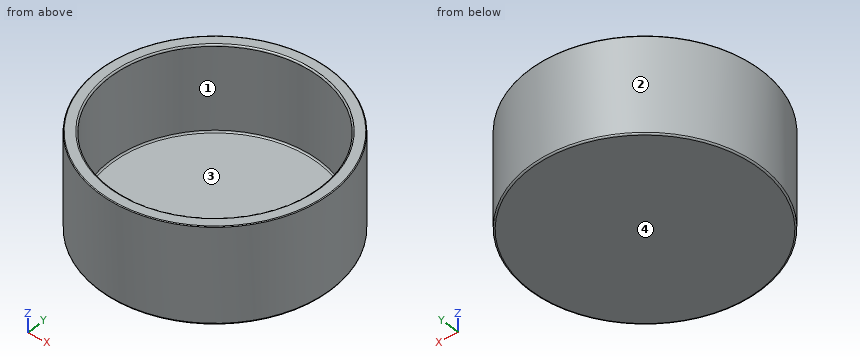
```python
from build123d import *

# Parameters (mm, degrees)
F0_R     = 31.25
F1_DEPTH = 3
F2_R     = 31.25
F2_R_2   = 28.25
F3_DEPTH = 23
F4_R     = 0.4
F5_R     = 0.2


with BuildPart() as f1:
    # F0 (on Top) → F1 (new body)
    with BuildSketch(Plane.XY):
        Circle(F0_R)
    extrude(amount=F1_DEPTH)

    # F2 (on face) → F3 (join)
    with BuildSketch(Plane.XY.offset(3)):
        Circle(F2_R)
        Circle(F2_R_2, mode=Mode.SUBTRACT)
    extrude(amount=F3_DEPTH)

    # F4
    f4_edges = [f1.edges().sort_by_distance(p)[0] for p in [
        (-28.25, 0, 26),
        (-28.25, 0, 3),
        (-31.25, 0, 0),
    ]]
    fillet(f4_edges, radius=F4_R)

    # F5
    f5_edges = [f1.edges().sort_by_distance(p)[0] for p in [
        (-31.25, 0, 26),
    ]]
    fillet(f5_edges, radius=F5_R)


solid = f1.part
```
The listing builds one solid part. Answer for the finished solid, in the listing's coordinates (mm). Face numbers are marked on the shaded views. Give positions to 0.01 mm unless a question says otherwise; leave off trailing zeros. Order: outer loops, then holes, each group sorted by start corner. A loop starts at its lowest first (then second) coordinate and runs counter-clockwise, first axis right, second up. Notation, with made-up numbers: (-4.75, 61.25) - (21.25, 61.25) arc R22 cw to (21.25, 84.25) - close; hole circle Ø2 at (88, 7.5). An arc over 180 degrees is marked (long way). Answer in a Markdown table with one row per item. Add a question column.
Q1. Given P1, Ø1.5, axis at y = 15.5, z = 6.5, coming from the -X side; P2, Ø10, axis at y = -16, z = 16.5, coming from the -X side; P3, Ø1, axis at y = 15, z = 17.5, coming from the -X side, each flat-ended and moving along its own axis, determine where each tip first touches the part or whether it passes through.
Q2. The part is cut by section A-A (y = 0). Determine the outline of the cut face in (x, z), then the cut area to 3 significant figures.
Q3. The part is cut by section C-C (z = 21.25). Determine the outline of the cut face in (x, y).
Q4. Find the intervals of material crossed by line 1 along Y through (x, z) = (0, 14.5); line 2 along Z through (x, y) = (-19, -6); line 3 along X through (y, z) = (19, 19), in increasing order. Write a range as [from, to].
Q5. For a pull along X with two mould halves and no side action, classify the marked faces 1, 2, 3 and 4 as released by +X, released by -X, zero draft, split by the parting line, or undercut.
Determined:
| question | item | result |
|---|---|---|
| 1 | P1 | stops at x = -27.55 |
| 1 | P2 | stops at x = -29.25 |
| 1 | P3 | stops at x = -27.68 |
| 2 | outline | (-31.25, 0.4) arc R0.4 ccw to (-30.85, 0) - (30.85, 0) arc R0.4 ccw to (31.25, 0.4) - (31.25, 25.8) arc R0.2 ccw to (31.05, 26) - (28.65, 26) arc R0.4 ccw to (28.25, 25.6) - (28.25, 3.4) arc R0.4 cw to (27.85, 3) - (-27.85, 3) arc R0.4 cw to (-28.25, 3.4) - (-28.25, 25.6) arc R0.4 ccw to (-28.65, 26) - (-31.05, 26) arc R0.2 ccw to (-31.25, 25.8) - close |
| 2 | area | 325 mm² |
| 3 | outline | circle Ø62.5 at (0, 0); hole circle Ø56.5 at (0, 0) |
| 4 | line 1 | y = [-31.25, -28.25], [28.25, 31.25] |
| 4 | line 2 | z = [0, 3] |
| 4 | line 3 | x = [-24.81, -20.91], [20.91, 24.81] |
| 5 | face 1 | undercut |
| 5 | face 2 | split by the parting line |
| 5 | face 3 | undercut |
| 5 | face 4 | zero draft |
